Build history of the part. All positions in model axes, mm. Give positions to 0.01 mm unless a question says otherwise; leave off trailing zeros. Order: outer loops, then holes, each group sorted by start corner. A loop starts at its lowest first (then second) coordinate and runs counter-clockwise, first axis right, second up. Notation, with made-up numbers: M 76.5,38.5 L 92.5,38.5 A22 cw 92.5,47.5 Z; hole C 4,69.25 d1. An arc over 180 degrees is marked long. Answer as CSV lines item,"result".
from build123d import *

# Parameters (mm, degrees)
SKETCH1_W               = 200
SKETCH1_H               = 100
BOSS_EXTRUDE1_DEPTH     = 2.6
FILLET1_R               = 10
SKETCH6_R               = 1.5
CUT_EXTRUDE6_DEPTH      = 2.6
MIRROR6_COPY_1_SKETCH_R = 1.5
MIRROR6_COPY_1_DEPTH    = 2.6
SKETCH15_R              = 10
CUT_EXTRUDE14_DEPTH     = 224.621913059
SKETCH23_R              = 1.524
CUT_EXTRUDE16_DEPTH     = 2.59999988
MIRROR8_COPY_1_SKETCH_R = 1.524
MIRROR8_COPY_1_DEPTH    = 2.59999988


with BuildPart() as part:
    # Sketch1 → Boss-Extrude1 (new body)
    with BuildSketch(Plane(origin=(0, 0, 0), x_dir=(1, 0, 0), z_dir=(0, 1, 0))):
        with Locations((100, -50)):
            Rectangle(SKETCH1_W, SKETCH1_H)
    extrude(amount=BOSS_EXTRUDE1_DEPTH)

    # Fillet1
    fillet1_edges = [part.edges().sort_by_distance(p)[0] for p in [
        (0, 1.3, 0),
        (200, 1.3, 0),
        (200, 1.3, 100),
        (0, 1.3, 100),
    ]]
    fillet(fillet1_edges, radius=FILLET1_R)

    # Sketch6 → Cut-Extrude6 (cut)
    with BuildSketch(Plane.XZ):
        with Locations(Location((190, 10, 0), (0, 0, 270))):
            Circle(SKETCH6_R)
    cut_extrude6 = extrude(amount=-CUT_EXTRUDE6_DEPTH, mode=Mode.SUBTRACT)

    # Mirror5: Cut-Extrude6 across plane
    add(cut_extrude6.mirror(Plane(origin=(100, 0, 0), x_dir=(0, 0, 1), z_dir=(1, 0, 0))), mode=Mode.SUBTRACT)

    # Mirror6: Cut-Extrude6 across plane
    add(cut_extrude6.mirror(Plane.XY.offset(50)), mode=Mode.SUBTRACT)

    # Mirror6 copy 1 sketch → Mirror6 copy 1 (cut)
    with BuildSketch(Plane(origin=(200, 0, 100), x_dir=(-1, 0, 0), z_dir=(0, -1, 0))):
        with Locations(Location((190, 10, 0), (0, 0, 270))):
            Circle(MIRROR6_COPY_1_SKETCH_R)
    extrude(amount=-MIRROR6_COPY_1_DEPTH, mode=Mode.SUBTRACT)

    # Sketch15 → Cut-Extrude14 (cut, through all)
    with BuildSketch(Plane.XZ):
        with Locations(Location((100, 50, 0), (0, 0, 270))):
            Circle(SKETCH15_R)
    extrude(amount=-CUT_EXTRUDE14_DEPTH, mode=Mode.SUBTRACT)

    # Sketch23 → Cut-Extrude16 (cut)
    with BuildSketch(Plane(origin=(0, 2.6, 0), x_dir=(1, 0, 0), z_dir=(0, 1, 0))):
        with Locations(Location((19.812, -9.906, 0), (0, 0, 270))):
            Circle(SKETCH23_R)
    cut_extrude16 = extrude(amount=-CUT_EXTRUDE16_DEPTH, mode=Mode.SUBTRACT)

    # Mirror7: Cut-Extrude16 across plane
    add(cut_extrude16.mirror(Plane(origin=(100, 0, 0), x_dir=(0, 0, 1), z_dir=(1, 0, 0))), mode=Mode.SUBTRACT)

    # Mirror8: Cut-Extrude16 across plane
    add(cut_extrude16.mirror(Plane.XY.offset(50)), mode=Mode.SUBTRACT)

    # Mirror8 copy 1 sketch → Mirror8 copy 1 (cut)
    with BuildSketch(Plane(origin=(200, 2.6, 100), x_dir=(-1, 0, 0), z_dir=(0, 1, 0))):
        with Locations(Location((19.812, -9.906, 0), (0, 0, 270))):
            Circle(MIRROR8_COPY_1_SKETCH_R)
    extrude(amount=-MIRROR8_COPY_1_DEPTH, mode=Mode.SUBTRACT)


solid = part.part
Item 1: Drop a flat-ended pin along its axis: pin 1 (5 mm diameter, centred on x = 10, z = 90, fed in from -Y). Give the stop position or say it passes through.
Geometry says:
pin 1,"stops at y = 0"
Item 2: Probe line 1 along Z through (x, y) = (190, 0.5); line 2 along X through (y, z) = (1.65, 10); line 3 along X through (y, z) = (1.3, 50). List the from-to ranges inside material, lowest first. Write a range as from..to.
Geometry says:
line 1,"z = 0..8.5, 11.5..88.5, 91.5..100"
line 2,"x = 0..8.5, 11.5..18.29, 21.33..178.67, 181.71..188.5, 191.5..200"
line 3,"x = 0..90, 110..200"
Item 3: Band-saw the part on C-C (y = 1.85). State how many separate pieces and enclosed holes the cut face has, and give its area (3 significant figures).
Geometry says:
separate pieces,"1"
enclosed holes,"9"
area,"19,500 mm2"
Item 4: Band-saw the part on A-A (z = 50). Give the cut face in (x, y), and give its area (3 significant figures).
Geometry says:
outline,"M 0,0 L 90,0 L 90,2.6 L 0,2.6 Z; M 110,0 L 200,0 L 200,2.6 L 110,2.6 Z"
area,"468 mm2"
Item 5: Band-saw the part on B-B (x = 100). Give the cut face in (y, z), and give its area (3 significant figures).
Geometry says:
outline,"M 0,0 L 2.6,0 L 2.6,40 L 0,40 Z; M 0,60 L 2.6,60 L 2.6,100 L 0,100 Z"
area,"208 mm2"
Item 6: Pull direction Z, two halves, no side cores. Call faces 1 (the cylindrical face through (109.915, 1.282, 51.302)), 2 (the cylindrical face through (2.85, 1.32, 96.99)), 3 (the flat face through (99, 0, 38)): released by +Z, released by -Z, zero draft, split by the parting line, or undercut.
Geometry says:
face 1,"undercut"
face 2,"released by +Z"
face 3,"zero draft"
